Autodesk Inventor part; units mm, degrees
ref_plane "YZ Plane" through (0, 0, 0) normal (1, 0, 0) x (0, 1, 0)
ref_plane "XZ Plane" through (0, 0, 0) normal (0, 1, 0) x (-1, 0, 0)
ref_plane "XY Plane" through (0, 0, 0) normal (0, 0, 1) x (1, 0, 0)
sketch "Sketch1" plane through (0, 0, 0) normal (0, 1, 0) x (-1, 0, 0)
  line L0 (0, 0) -> (10, 0)
  circle A0 centre (10, 0) radius 1.5
  line L1 (0, 0) -> (-10, 0)
  circle A1 centre (-10, 0) radius 1.5
  line L2 (0, 0) -> (0, 6)
  line L3 (0, 6) -> (15, 6)
  line L4 (15, 6) -> (15, 16)
  line L5 (15, 16) -> (-15, 16)
  line L6 (-15, 16) -> (-15, 6)
  line L7 (-15, 6) -> (0, 6)
  dimension "d0" = 10
  dimension "d1" = 3
  dimension "d2" = 10
  dimension "d3" = 3
  dimension "d4" = 6
  dimension "d5" = 15
  dimension "d7" = 10
  dimension "d8" = 30
  dimension "d9" = 10
extrude "Extrusion1" add sketch "Sketch1" along normal blind 5 contours L7 L6 L5 L4 L3
fillet "Fillet1" radius 5 2 edges at (-7.5, 5, 6) (0, 5, 16)
sketch "Sketch2" plane through (0, 0, 0) normal (0, -1, 0) x (1, 0, 0)
  line L0 (0, 0) -> (0, -5)
  line L1 (0, -5) -> (-25, -5)
  line L2 (-25, -5) -> (-25, 25)
  line L3 (-25, 25) -> (25, 25)
  line L4 (25, 25) -> (25, -5)
  line L5 (25, -5) -> (0, -5)
  dimension "d13" = 5
  dimension "d14" = 25
  dimension "d15" = 30
  dimension "d16" = 50
  dimension "d17" = 30
extrude "Extrusion2" add sketch "Sketch2" along normal blind 70
sketch "Sketch3" plane through (-25, 0, 25) normal (0, 0, 1) x (1, 0, 0)
  line L0 (0, 0) -> (0, -70)
  line L1 (0, 0) -> (0, -20)
  line L2 (0, -20) -> (50, -20)
  line L3 (50, 0) -> (50, -70)
  line L4 (50, -20) -> (50, -10)
  line L5 (50, -10) -> (0, -10)
  point P0 (25, 0)
  dimension "d20" = 20
  dimension "d21" = 10
extrude "Extrusion3" add sketch "Sketch3" along normal blind 225
sketch "Sketch4" plane through (-25, -20, 25) normal (0, -1, 0) x (1, 0, 0)
  line L0 (50, 0) -> (50, 225)
  line L1 (50, 225) -> (50, 200)
  line L2 (50, 200) -> (0, 200)
  line L3 (0, 0) -> (0, 225)
  line L4 (0, 225) -> (0, 200)
  line L5 (0, 225) -> (50, 225)
  point P0 (25, -25)
  dimension "d24" = 25
extrude "Extrusion4" add sketch "Sketch4" along normal blind 50
properties part number "carSpacer"
For this review, take the finished solid that the model builds, in its own axes (mm). A direction names the side the tool comes from. Coordinates: 2 decimals unless noted, no trailing zeros. Write each loop counter-clockwise with the first axis right and the second up, starting at its lowest first coordinate (ties: lowest second). Pieces come first, ordered by that corner, then holes.
(1) For pin 1 Ø3 at (x, z) = (14, 191) entering from -Y; pin 2 Ø8 at (x, z) = (18.5, 217.5) entering from +Y; pin 3 Ø8 at (x, y) = (4, -4.5) entering from +Z, all flat-tipped, find the tip position at first contact; note any pin that passes through.
(2) The part is to be moulded in two halves that separate along Z. For faces 1 (the face through (0, -40, 250)), 2 (the face through (0, -45, 25)), 3 (the face through (25, -19, 121)), 4 (the face through (0, -45, 225)), say which applies: +Z half, -Z half, draft (parallel to the pull), parting line (faces both ways), or undercut.
(3) Add section C-C on z = 147. Give the boundary of the cut face in (x, y), then the cut area to 3 significant figures.
(4) Add section B-B on x = 22. Give the boundary of the cut face in (y, z).
(5) Wall thickness on probe 1 along Z at (x, y) = (-11, -58.5); probe 2 along Y at (x, z) = (-6.5, 198); probe 3 along Y at (x, z) = (15, 237): over which ranges is each line inside the solid? List them lowest first.
(6) Add section A-A on y = -23. Give the boundary of the cut face in (x, z).
(7) Tool access review of faces 5 (the face through (-15, 2, 11)), 6 (the face through (0, -20, 124)), 7 (the face through (15, 2, 11)), 8 (the face through (0, -5, 25)): name each direction out of +Z, -Z, +X, -X, +Y, -Y from which nothing blocks a thin tool from reaching the whole face with its end or side.
Answer sheet:
1. pin 1: stops at y = -20
1. pin 2: stops at y = -10
1. pin 3: stops at z = 25
2. face 1: +Z half
2. face 2: undercut
2. face 3: draft
2. face 4: undercut
3. outline: (-25, -20) - (25, -20) - (25, -10) - (-25, -10) - close
3. area: 500 mm2
4. outline: (-70, -5) - (0, -5) - (0, 25) - (-10, 25) - (-10, 250) - (-70, 250) - (-70, 225) - (-20, 225) - (-20, 25) - (-70, 25) - close
5. probe 1: z = -5 to 25, 225 to 250
5. probe 2: y = -20 to -10
5. probe 3: y = -70 to -10
6. outline: (-25, -5) - (25, -5) - (25, 25) - (-25, 25) - close; (-25, 225) - (25, 225) - (25, 250) - (-25, 250) - close
7. face 5: +Z, -Z, -X, +Y
7. face 6: +X, -X, -Y
7. face 7: +Z, -Z, +X, +Y
7. face 8: +Z, +X, -X, +Y
